Geometry check sheet. Reference: the model listing, model coordinates, mm. A direction names the side the tool comes from. Round coordinates to 2 decimals unless told otherwise and drop trailing zeros. Order: outer loops, then holes, each group sorted by start corner. A loop starts at its lowest first (then second) coordinate and runs counter-clockwise, first axis right, second up. Notation, with made-up numbers: (86.25, -17.75) - (127.25, -17.75) arc R16 ccw to (127.25, 7.25) - close; hole circle Ø8 at (-38.5, -31.5). An arc over 180 degrees is marked (long way). Use a Markdown table: item, result. Add a question column.
(1) Section check B-B on x = 0. Record the boundary of the cut face in (y, z), then the cut area to 3 significant figures.
(2) Section check A-A on z = 0. Record the boundary of the cut face in (x, y).
(3) Access from +Z, -Z, +X, -X, +Y, -Y to the whole of each face (thin tool, end or side, straight path). Record for faces 4 (the face through (-1.08, 17.03, 4.88)), 5 (the face through (2, -15, 2)), 6 (the face through (-0.54, -0.21, 2.44)).
(4) Thickness scan on line 1 along Z through (x, y) = (0, 16); line 2 along Z through (x, y) = (0, -7.25). Record the ranges inside material, lowest first. Write a range as [from, to].
(5) Mould release check, pull along X, two halves, no side actions. Record for faces 1 (the face through (2, -19, 5)), 2 (the face through (-5.158, 0.266, 3.955)), 3 (the face through (2, 15, 2)): released by +X, released by -X, zero draft, split by the parting line, or undercut.
(6) Section check D-D on x = 3. Record the boundary of the cut face in (y, z).
(7) Gauge pin test, flat ends, axial feed: P1, Ø3, axis at x = -3.5, z = -0.5, coming from the -Y side; P2, Ø3, axis at x = 4, y = -11, coming from the -Z side; P3, Ø1, axis at x = -3, y = 3.5, coming from the +Z side; P4, Ø1.5, axis at y = 12, z = 3, coming from the +X side. Record the tip position at first contact, or that the pin passes through.
(8) Section check C-C on y = 13.5. Record the boundary of the cut face in (x, z).
```python
from build123d import *

# Parameters (mm, degrees)
SKETCH_1_R          = 6.5
SKETCH_1_R_2        = 2.5
EXTRUDE_2_DEPTH     = 19
SKETCH_2_R          = 5
CUT_EXTRUDE_1_DEPTH = 4


with BuildPart() as part:
    # 草图1 → 凸台-拉伸2 (new body, symmetric)
    with BuildSketch(Plane(origin=(0, 0, 0), x_dir=(1, 0, 0), z_dir=(0, 1, 0))):
        Circle(SKETCH_1_R)
        Circle(SKETCH_1_R_2, mode=Mode.SUBTRACT)
    extrude(amount=EXTRUDE_2_DEPTH, both=True)

    # 草图2 → 切除-拉伸1 (cut)
    with BuildSketch(Plane(origin=(0, 19, 0), x_dir=(1, 0, 0), z_dir=(0, 1, 0))):
        Circle(SKETCH_2_R)
    cut_extrude_1 = extrude(amount=-CUT_EXTRUDE_1_DEPTH, mode=Mode.SUBTRACT)

    # 镜向1: 切除-拉伸1 across plane
    add(cut_extrude_1.mirror(Plane.ZX), mode=Mode.SUBTRACT)


solid = part.part
```
Check sheet entries:
| question | item | result |
|---|---|---|
| 1 | outline | (-19, -6.5) - (19, -6.5) - (19, -5) - (15, -5) - (15, -2.5) - (-15, -2.5) - (-15, -5) - (-19, -5) - close; (-19, 5) - (-15, 5) - (-15, 2.5) - (15, 2.5) - (15, 5) - (19, 5) - (19, 6.5) - (-19, 6.5) - close |
| 1 | area | 264 mm2 |
| 2 | outline | (-6.5, -19) - (-5, -19) - (-5, -15) - (-2.5, -15) - (-2.5, 15) - (-5, 15) - (-5, 19) - (-6.5, 19) - close; (2.5, -15) - (5, -15) - (5, -19) - (6.5, -19) - (6.5, 19) - (5, 19) - (5, 15) - (2.5, 15) - close |
| 3 | face 4 | +Y |
| 3 | face 5 | -Y |
| 3 | face 6 | +Y, -Y |
| 4 | line 1 | z = [-6.5, -5], [5, 6.5] |
| 4 | line 2 | z = [-6.5, -2.5], [2.5, 6.5] |
| 5 | face 1 | zero draft |
| 5 | face 2 | split by the parting line |
| 5 | face 3 | undercut |
| 6 | outline | (-19, -5.77) - (19, -5.77) - (19, -4) - (15, -4) - (15, 4) - (19, 4) - (19, 5.77) - (-19, 5.77) - (-19, 4) - (-15, 4) - (-15, -4) - (-19, -4) - close |
| 7 | P1 | stops at y = -19 |
| 7 | P2 | stops at z = -6 |
| 7 | P3 | stops at z = 6 |
| 7 | P4 | stops at x = 6.1 |
| 8 | outline | circle Ø13 at (0, 0); hole circle Ø5 at (0, 0) |
